from build123d import *

# Parameters (mm, degrees)
F0_W     = 12.7
F0_H     = 12.7
F1_DEPTH = 50.8
F2_SIZE  = 10.16
F3_SIZE  = 10.16
F4_R     = 7.770906
F5_DEPTH = 99.568


with BuildPart() as f1:
    # F0 (on Front) → F1 (new body)
    with BuildSketch(Plane.XZ):
        with Locations((37.287199, -32.969202)):
            Rectangle(F0_W, F0_H)
        with Locations((-91.128487, -32.969202)):
            Rectangle(F0_W, F0_H)
        Polygon((-84.778487, -26.619202), (-84.778487, -39.319202), (-58.57092, -39.319202), (-58.57092, -23.7744), (5.334001, -23.7744), (5.334001, -39.319202), (30.937199, -39.319202), (30.937199, -26.619202), (18.3388, -26.619202), (18.3388, 32.613602), (-7.0612, 32.613602), (-7.0612, -13.1064), (-45.1612, -13.1064), (-45.1612, 32.613602), (-70.5612, 32.613602), (-70.5612, -26.619202), align=None)
    extrude(amount=F1_DEPTH)

    # F2
    f2_edges = [f1.edges().sort_by_distance(p)[0] for p in [
        (43.637199, -50.8, -32.969202),
    ]]
    chamfer(f2_edges, length=F2_SIZE)

    # F3
    f3_edges = [f1.edges().sort_by_distance(p)[0] for p in [
        (-97.478487, -50.8, -32.969202),
    ]]
    chamfer(f3_edges, length=F3_SIZE)

    # F4 (on face) → F5 (cut)
    with BuildSketch(Plane.YZ.offset(18.3388)):
        with Locations((-25.755601, 13.411201)):
            Circle(F4_R)
    extrude(amount=-F5_DEPTH, mode=Mode.SUBTRACT)


solid = f1.part
CAD build for the part. Positions are in the model's coordinates, mm. A direction names the side the tool comes from. Coordinates: 2 decimals unless noted, no trailing zeros. Write each loop counter-clockwise with the first axis right and the second up, starting at its lowest first coordinate (ties: lowest second). Pieces come first, ordered by that corner, then holes. Notation, with made-up numbers: (18.25, 87) - (25.25, 87) arc R38 ccw to (25.25, 126) - close; hole circle Ø10 at (-37.75, -15). An arc over 180 degrees is marked (long way). Use a Markdown table: item, result. Add a question column.
Item 1: Band-saw the part on C-C, the plane y = -22. Give the cut face in (x, z), and give its area (3 significant figures).
Item 2: Drill centre lines: L1, parallel to X at y = -44.5, z = 0; L2, parallel to Z at x = -14, y = -40; L3, parallel to X at y = -37.5, z = -28. Where is each one in solid material? Low to high. Write a range as from..to.
Item 3: Band-saw the part on A-A, the plane z = -7.5. Give the cut face in (x, y), and give its area (3 significant figures).
Item 4: Band-saw the part on D-D, the plane x = -9. Give the cut face in (y, z).
Item 5: Band-saw the part on B-B, the plane y = -35.5. Give the cut face in (x, z), and give its area (3 significant figures).
Item 6: Mould opens along Y. For faces 6 (the face through (-58.571, -25, -32)), 7 (the face through (-27, 0, -14)), 8 (the face through (-57.683, -31.483, 18.663)) say: pulls with the +Y half, pulls with the -Y half, needs draft (parallel to the pull), parting line crosses it, or undercut.
Item 7: Flat gauge pins, fed straight in: pin 1 (15 mm diameter, centred on y = -35.5, z = 17.5, fed in from -X); pin 2 (14 mm diameter, centred on y = -25.76, z = 13.41, fed in from +X); pin 3 (4 mm diameter, centred on x = -54.5, y = -29.5, fed in from -Z); pin 4 (2 mm diameter, centred on x = -25.5, y = -17, fed in from +Z). Where does each tip first touch, or does it go through?
Item 8: 3-axis set-ups, long thin cutter, end or side, ignore diameter. For faces 1 (the face through (5.817, -31.483, 18.663)), 2 (the face through (31, -25, -26.619)), 3 (the face through (5.334, -25, -31)), 4 (the face through (-70.561, -25, 3)), 5 (the face through (-7.061, -25, 5)): which of +Z, -Z, +X, -X, +Y, -Y reach the whole face in a straight line?
Numbers:
| question | item | result |
|---|---|---|
| 1 | outline | (-97.48, -39.32) - (-58.57, -39.32) - (-58.57, -23.77) - (5.33, -23.77) - (5.33, -39.32) - (43.64, -39.32) - (43.64, -26.62) - (18.34, -26.62) - (18.34, 6.61) - (-7.06, 6.61) - (-7.06, -13.11) - (-45.16, -13.11) - (-45.16, 6.61) - (-70.56, 6.61) - (-70.56, -26.62) - (-97.48, -26.62) - close; (-70.56, 20.21) - (-45.16, 20.21) - (-45.16, 32.61) - (-70.56, 32.61) - close; (-7.06, 20.21) - (18.34, 20.21) - (18.34, 32.61) - (-7.06, 32.61) - close |
| 1 | area | 3,630 mm2 |
| 2 | L1 | -70.56..-45.16, -7.06..18.34 |
| 2 | L2 | -23.77..-13.11 |
| 2 | L3 | -97.48..-58.57, 5.33..43.64 |
| 3 | outline | (-70.56, -50.8) - (-45.16, -50.8) - (-45.16, 0) - (-70.56, 0) - close; (-7.06, -50.8) - (18.34, -50.8) - (18.34, 0) - (-7.06, 0) - close |
| 3 | area | 2,580 mm2 |
| 4 | outline | (-50.8, -23.77) - (0, -23.77) - (0, -13.11) - (-50.8, -13.11) - close |
| 5 | outline | (-97.48, -39.32) - (-58.57, -39.32) - (-58.57, -23.77) - (5.33, -23.77) - (5.33, -39.32) - (43.64, -39.32) - (43.64, -26.62) - (18.34, -26.62) - (18.34, 32.61) - (-7.06, 32.61) - (-7.06, -13.11) - (-45.16, -13.11) - (-45.16, 32.61) - (-70.56, 32.61) - (-70.56, -26.62) - (-97.48, -26.62) - close |
| 5 | area | 4,320 mm2 |
| 6 | face 6 | needs draft |
| 6 | face 7 | pulls with the +Y half |
| 6 | face 8 | undercut |
| 7 | pin 1 | x = -70.56 |
| 7 | pin 2 | through |
| 7 | pin 3 | z = -23.77 |
| 7 | pin 4 | z = -13.11 |
| 8 | face 1 | +X, -X |
| 8 | face 2 | +Z, +X, +Y, -Y |
| 8 | face 3 | -Z, +Y, -Y |
| 8 | face 4 | +Z, -X, +Y, -Y |
| 8 | face 5 | +Z, +Y, -Y |
